from build123d import *
from build123d.topology import SkipClean

# Parameters (mm, degrees)
SKETCH1_R           = 38
BOSS_EXTRUDE1_DEPTH = 5
SKETCH1_4_R         = 34.75
BOSS_EXTRUDE2_DEPTH = 10
THREAD1_PITCH       = 4
SKETCH6_R           = 32.750011187
CUT_EXTRUDE1_DEPTH  = 10


with BuildPart() as part:
    # Sketch1 → Boss-Extrude1 (new body)
    with BuildSketch(Plane(origin=(0, 0, 0), x_dir=(1, 0, 0), z_dir=(0, 1, 0))):
        with Locations(Location((0, 0, 0), (0, 0, 270))):
            Circle(SKETCH1_R)
    extrude(amount=-BOSS_EXTRUDE1_DEPTH)

    # Sketch1<4> → Boss-Extrude2 (add)
    with BuildSketch(Plane(origin=(0, 0, 0), x_dir=(1, 0, 0), z_dir=(0, 1, 0))):
        with Locations(Location((0, 0, 0), (0, 0, 270))):
            Circle(SKETCH1_4_R)
    extrude(amount=BOSS_EXTRUDE2_DEPTH)

    # Thread1: the profile of Thread Profile1 profile screwed along a right-hand helix of 2.5 turns, 12 arcs to a turn; built about Z, then put on its axis
    thread1_z = Axis((0, 0, 0), (0, 0, 1))
    thread1_corners = [(34.7497, 0, -0.000173205), (36.9150635, 0, 1.249999995), (36.9150635, 0, 1.749999995), (34.7497, 0, 3.000173194)]
    with BuildLine(mode=Mode.PRIVATE) as thread1_profile:
        Line(thread1_corners[0], thread1_corners[1])
        Line(thread1_corners[1], thread1_corners[2])
        Line(thread1_corners[2], thread1_corners[3])
        Line(thread1_corners[3], thread1_corners[0])
    thread1_cap = Face(thread1_profile.wire())
    thread1_turn_angles = [0, 15, 30, 45, 60, 75, 90, 105, 120, 135, 150, 165, 180, 195, 210, 225, 240, 255, 270, 285, 300, 315, 330, 345, 360]
    thread1_turn_weights = [1, 0.9659258262890683, 1, 0.9659258262890683, 1, 0.9659258262890683, 1, 0.9659258262890683, 1, 0.9659258262890683, 1, 0.9659258262890683, 1, 0.9659258262890683, 1, 0.9659258262890683, 1, 0.9659258262890683, 1, 0.9659258262890683, 1, 0.9659258262890683, 1, 0.9659258262890683, 1]
    thread1_turn_rails = [Edge.make_bspline([Vector(p[0], p[1], 0).rotate(thread1_z, thread1_turn_angles[k]) / thread1_turn_weights[k] + Vector(0, 0, p[2] + THREAD1_PITCH * thread1_turn_angles[k] / 360) for k in range(25)], [0, 0, 0, 1, 1, 2, 2, 3, 3, 4, 4, 5, 5, 6, 6, 7, 7, 8, 8, 9, 9, 10, 10, 11, 11, 12, 12, 12], 2, thread1_turn_weights) for p in thread1_corners]
    thread1_turn_sides = [Face.make_surface_from_curves(thread1_turn_rails[p[0]], thread1_turn_rails[p[1]]) for p in [(0, 1), (1, 2), (2, 3), (3, 0)]]
    thread1_last_angles = [720, 735, 750, 765, 780, 795, 810, 825, 840, 855, 870, 885, 900]
    thread1_last_weights = [1, 0.9659258262890683, 1, 0.9659258262890683, 1, 0.9659258262890683, 1, 0.9659258262890683, 1, 0.9659258262890683, 1, 0.9659258262890683, 1]
    thread1_last_rails = [Edge.make_bspline([Vector(p[0], p[1], 0).rotate(thread1_z, thread1_last_angles[k]) / thread1_last_weights[k] + Vector(0, 0, p[2] + THREAD1_PITCH * thread1_last_angles[k] / 360) for k in range(13)], [0, 0, 0, 1, 1, 2, 2, 3, 3, 4, 4, 5, 5, 6, 6, 6], 2, thread1_last_weights) for p in thread1_corners]
    thread1_last_sides = [Face.make_surface_from_curves(thread1_last_rails[p[0]], thread1_last_rails[p[1]]) for p in [(0, 1), (1, 2), (2, 3), (3, 0)]]
    thread1 = Plane(origin=(0, 10, 0), x_dir=(-1, 0, 0), z_dir=(0, -1, 0)) * Solid(Shell([*[p.moved(Location((0, 0, THREAD1_PITCH * i))) for i in range(2) for p in thread1_turn_sides], *thread1_last_sides, thread1_cap, thread1_cap.rotate(thread1_z, 900).moved(Location((0, 0, THREAD1_PITCH * 900 / 360)))]))
    add(thread1)

    # Sketch6 → Cut-Extrude1 (cut)
    with SkipClean():  # the faces are left unmerged after this step: merging them gives an invalid solid
        with BuildSketch(Plane(origin=(0, 10, 0), x_dir=(1, 0, 0), z_dir=(0, 1, 0))):
            with Locations(Location((0, 0, 0), (0, 0, 270))):
                Circle(SKETCH6_R)
        extrude(amount=-CUT_EXTRUDE1_DEPTH, mode=Mode.SUBTRACT)


solid = part.part
CAD build for the part. Positions are in the model's coordinates, mm. A direction names the side the tool comes from. Coordinates: 2 decimals unless noted, no trailing zeros. Write each loop counter-clockwise with the first axis right and the second up, starting at its lowest first coordinate (ties: lowest second). Pieces come first, ordered by that corner, then holes. Notation, with made-up numbers: M -2,86.25 L 30,86.25 A26 cw 30,105.25 Z; hole C 73,60 d8. An arc over 180 degrees is marked long. Answer as a JSON object with one key per item and string values. Group by question number.
1) Pin check, flat tips, straight feed: pin 1 Ø6 at (y, z) = (-1, 16.5) entering from +X; pin 2 Ø6 at (x, y) = (20, 1.5) entering from -Z; pin 3 Ø1 at (y, z) = (2, 7.5) entering from -X. Stop position of each tip, or through.
2) Wall check: line 1 (X direction, y = 6.5, z = 0); line 2 (Z direction, x = -1, y = 7.5); line 3 (Y direction, x = 15.5, z = -20.5). Give the ranges that are in metal, low to high. Write a range as from..to.
3) Mould opens along Y. For faces 3 (the face through (1, -5, -1)), 4 (the face through (0, 0, 0)), 5 (the face through (31, 0, 17)), 6 (the face through (-31.97, 5.07, -7.1)) say: +Y half, -Y half, draft (parallel to the pull), parting line (faces both ways), or undercut.
4) Saw through at A-A (y = -1.5). Write the cut outline in (x, z).
5) Tool access for faces 1 (the face through (-36, 8, 0)), 2 (the face through (23.3, 10, -23.3)): list every direction of +Z, -Z, +X, -X, +Y, -Y with a clear straight run to the whole face (end or side of a thin tool).
Values follow:
{
 "1": {"pin 1": "stops at x = 35.52", "pin 2": "stops at z = -33.78", "pin 3": "stops at x = -35.06"},
 "2": {"line 1": "x = -34.75..-32.75, 32.75..36.92", "line 2": "z = -36.9..-32.73, 32.73..34.74", "line 3": "y = -5..0"},
 "3": {"face 3": "-Y half", "face 4": "+Y half", "face 5": "undercut", "face 6": "draft"},
 "4": {"outline": "C 0,0 d76"},
 "5": {"face 1": "+Z, -X, +Y", "face 2": "+Z, -Z, +X, -X, +Y"}
}
